from build123d import *

# Parameters (mm, degrees)
SKETCH_1_W      = 98.5
SKETCH_1_H      = 18.5
SKETCH_1_R      = 1.6
EXTRUDE_1_DEPTH = 3
SKETCH_2_W      = 98.5
SKETCH_2_H      = 21.5
EXTRUDE_2_DEPTH = 3
FILLET_1_R      = 1
SKETCH_3_W      = 98.5
SKETCH_3_H      = 3
EXTRUDE_3_DEPTH = 9


with BuildPart() as part:
    # 草图1 → 凸台-拉伸1 (new body)
    with BuildSketch(Plane.XY):
        with Locations((0, 9.25)):
            Rectangle(SKETCH_1_W, SKETCH_1_H)
        with Locations((-46.25, 3)):
            Circle(SKETCH_1_R, mode=Mode.SUBTRACT)
        with Locations((-46.25, 9.5)):
            Circle(SKETCH_1_R, mode=Mode.SUBTRACT)
        with Locations((46.25, 3)):
            Circle(SKETCH_1_R, mode=Mode.SUBTRACT)
        with Locations((46.25, 9.5)):
            Circle(SKETCH_1_R, mode=Mode.SUBTRACT)
    extrude(amount=EXTRUDE_1_DEPTH)

    # 草图2 → 凸台-拉伸2 (add)
    with BuildSketch(Plane(origin=(0, 18.5, 0), x_dir=(1, 0, 0), z_dir=(0, 1, 0))):
        with Locations((0, -13.75)):
            Rectangle(SKETCH_2_W, SKETCH_2_H)
    extrude(amount=-EXTRUDE_2_DEPTH)

    # 圆角1
    fillet_1_edges = [part.edges().sort_by_distance(p)[0] for p in [
        (0, 15.5, 3),
        (0, 18.5, 0),
    ]]
    fillet(fillet_1_edges, radius=FILLET_1_R)

    # 草图3 → 凸台-拉伸3 (add)
    with BuildSketch(Plane.XZ):
        with Locations((0, 1.5)):
            Rectangle(SKETCH_3_W, SKETCH_3_H)
    extrude(amount=EXTRUDE_3_DEPTH)


solid = part.part
Build history of the part. All positions in model axes, mm. A direction names the side the tool comes from. Round coordinates to 2 decimals unless told otherwise and drop trailing zeros. Write each loop counter-clockwise with the first axis right and the second up, starting at its lowest first coordinate (ties: lowest second). Pieces come first, ordered by that corner, then holes. Notation, with made-up numbers: (21.25, 53) - (54.25, 53) arc R25 cw to (54.25, 85) - close; hole circle Ø11 at (11.25, 30.5). An arc over 180 degrees is marked (long way). Use CSV: the item, a comma, the result in double quotes.
(1) Band-saw the part on C-C (x = -23.5). Write the cut outline in (y, z), plus the area to 3 significant figures.
Response:
outline,"(-9, 0) - (17.5, 0) arc R1 ccw to (18.5, 1) - (18.5, 24.5) - (15.5, 24.5) - (15.5, 4) arc R1 cw to (14.5, 3) - (-9, 3) - close"
area,"147 mm²"
(2) Pin check, flat tips, straight feed: P1, Ø1.5, axis at x = 21.5, z = 10.5, coming from the -Y side; P2, Ø12, axis at x = -5, y = -0.5, coming from the +Z side. Stop position of each tip, or through.
Response:
P1,"y = 15.5"
P2,"z = 3"
(3) Band-saw the part on B-B (x = 46.25). Write the cut outline in (y, z), plus the area to 3 significant figures.
Response:
outline,"(-9, 0) - (1.4, 0) - (1.4, 3) - (-9, 3) - close; (4.6, 0) - (7.9, 0) - (7.9, 3) - (4.6, 3) - close; (11.1, 0) - (17.5, 0) arc R1 ccw to (18.5, 1) - (18.5, 24.5) - (15.5, 24.5) - (15.5, 4) arc R1 cw to (14.5, 3) - (11.1, 3) - close"
area,"128 mm²"
(4) 3-axis set-ups, long thin cutter, end or side, ignore diameter. For faces 1 (the cylindrical face through (46.99, 1.58, 1.48)), 2 (the flat face through (-1, 3, 3)): which of +Z, -Z, +X, -X, +Y, -Y reach the whole face in a straight line?
Response:
face 1,"+Z, -Z"
face 2,"+Z, +X, -X, -Y"
(5) Band-saw the part on D-D (z = 13.75). Write the cut outline in (x, y), plus the area to 4 significant figures.
Response:
outline,"(-49.25, 15.5) - (49.25, 15.5) - (49.25, 18.5) - (-49.25, 18.5) - close"
area,"295.5 mm²"
(6) Band-saw the part on A-A (y = 3). Write the cut outline in (x, z), plus the area to 3 significant figures.
Response:
outline,"(-49.25, 0) - (-47.85, 0) - (-47.85, 3) - (-49.25, 3) - close; (-44.65, 0) - (44.65, 0) - (44.65, 3) - (-44.65, 3) - close; (47.85, 0) - (49.25, 0) - (49.25, 3) - (47.85, 3) - close"
area,"276 mm²"
(7) Mould opens along Y. For faces 3 (the flat face through (-1, 17, 24.5)), 4 (the cylindrical face through (45.9, 7.94, 1.48)), 5 (the flat face through (-1, -9, 2)) say: pulls with the +Y half, pulls with the -Y half, needs draft (parallel to the pull), parting line crosses it, or undercut.
Response:
face 3,"needs draft"
face 4,"undercut"
face 5,"pulls with the -Y half"
(8) Wall check: line 1 (Y direction, x = -46.25, z = 1.65); line 2 (Z direction, x = -20.5, y = 2.75); line 3 (Y direction, x = -29, z = 4). Give the ranges that are in metal, low to high.
Response:
line 1,"-9 to 1.4, 4.6 to 7.9, 11.1 to 18.5"
line 2,"0 to 3"
line 3,"15.5 to 18.5"
